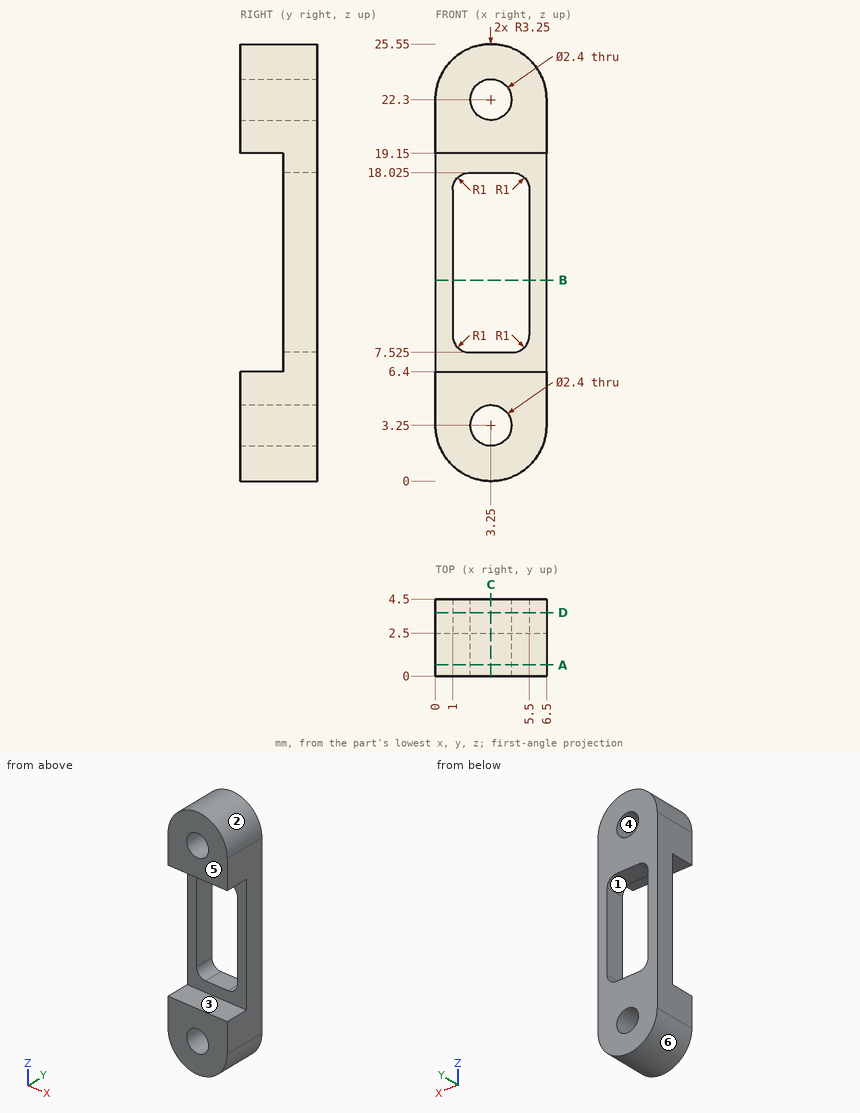
Geometry: see drawing. Coordinates: mm, zero at the bounding-box minimum. A direction names the side the tool comes from. Give positions to 0.01 mm unless a question says otherwise; leave off trailing zeros. Write each loop counter-clockwise with the first axis right and the second up, starting at its lowest first coordinate (ties: lowest second). Pieces come first, ordered by that corner, then holes. Notation, with made-up numbers: M 49.5,42.5 L 78.5,42.5 A9 cw 78.5,51.5 Z; hole C 43,-22 d10. An arc over 180 degrees is marked long. Answer in a Markdown table with one row per item. Add a question column.
(1) Reachability of the marked faces 1, 2 and 3 from +Z, -Z, +X, -X, +Y, -Y: full face, straight path, thin tool, end or side. Return the list, or none.
(2) Section D-D on y = 3.7. Return loops of the section in (x, z) (3 decimals).
(3) Section B-B on z = 11.75. Return loops of the section in (x, y).
(4) Section C-C on x = 3.25. Return loops of the section in (y, z) (3 decimals), and give its area (3 significant figures).
(5) First-contact query: pin 1 (1.4 mm diameter, centred on x = 3.25, z = 3.25, fed in from +Y); pin 2 (0.8 mm diameter, centred on x = 2, y = 2, fed in from +Z). Flat tips, straight axial feed; report the tip coordinate or a pass-through.
(6) Mould query, pull axis Z, two halves, no side actions, for the marked faces 4, 5 and 6. Classes: +Z half, -Z half, draft (parallel to the pull), parting line (faces both ways), or undercut.
(7) Ray query, line 1 (Z direction, x = 3.25, y = 1.15); line 2 (X direction, y = 2.65, z = 3.25); line 3 (Z direction, x = 4, y = 0.45). Return the intervals inside material, ascending.
(8) Section A-A on y = 0.65. Return loops of the section in (x, z), and give its area (3 significant figures).
Result set:
| question | item | result |
|---|---|---|
| 1 | face 1 | +Y, -Y |
| 1 | face 2 | +Z, +Y, -Y |
| 1 | face 3 | +X, -X, -Y |
| 2 | outline | M 0,3.25 A3.25 ccw 6.5,3.25 L 6.5,22.3 A3.25 ccw 0,22.3 Z; hole M 1,8.525 A1 ccw 2,7.525 L 4.5,7.525 A1 ccw 5.5,8.525 L 5.5,17.025 A1 ccw 4.5,18.025 L 2,18.025 A1 ccw 1,17.025 Z; hole C 3.25,3.25 d2.4; hole C 3.25,22.3 d2.4 |
| 3 | outline | M 0,2.5 L 1,2.5 L 1,4.5 L 0,4.5 Z; M 5.5,2.5 L 6.5,2.5 L 6.5,4.5 L 5.5,4.5 Z |
| 4 | outline | M 0,0 L 4.5,0 L 4.5,2.05 L 0,2.05 Z; M 0,4.45 L 4.5,4.45 L 4.5,7.525 L 2.5,7.525 L 2.5,6.4 L 0,6.4 Z; M 0,19.15 L 2.5,19.15 L 2.5,18.025 L 4.5,18.025 L 4.5,21.1 L 0,21.1 Z; M 0,23.5 L 4.5,23.5 L 4.5,25.55 L 0,25.55 Z |
| 4 | area | 40.5 mm^2 |
| 5 | pin 1 | passes through |
| 5 | pin 2 | stops at z = 25.44 |
| 6 | face 4 | undercut |
| 6 | face 5 | draft |
| 6 | face 6 | -Z half |
| 7 | line 1 | z = 0 to 2.05, 4.45 to 6.4, 19.15 to 21.1, 23.5 to 25.55 |
| 7 | line 2 | x = 0 to 2.05, 4.45 to 6.5 |
| 7 | line 3 | z = 0.09 to 2.31, 4.19 to 6.4, 19.15 to 21.36, 23.24 to 25.46 |
| 8 | outline | M 0,3.25 A3.25 ccw 6.5,3.25 L 6.5,6.4 L 0,6.4 Z; M 0,19.15 L 6.5,19.15 L 6.5,22.3 A3.25 ccw 0,22.3 Z; hole C 3.25,3.25 d2.4; hole C 3.25,22.3 d2.4 |
| 8 | area | 65.1 mm^2 |
